```python
from build123d import *

# Parameters (mm, degrees)
F0_W     = 355.6
F0_H     = 355.6
F1_DEPTH = 12.7
F2_W     = 355.6
F2_H     = 12.7
F4_DEPTH = 101.6
F5_W     = 330.2
F5_H     = 12.7
F6_DEPTH = 101.6


with BuildPart() as f1:
    # F0 (on Top) → F1 (new body)
    with BuildSketch(Plane.XY):
        Rectangle(F0_W, F0_H)
    extrude(amount=F1_DEPTH)

    # F2 (on face) + F3 (on face) → F4 (join)
    with BuildSketch(Plane.XY.offset(12.7)):
        with Locations((0, 171.45)):
            Rectangle(F2_W, F2_H)
    with BuildSketch(Plane.XY.offset(12.7)):
        Polygon((-165.1, -177.8), (-165.1, 177.8), (-177.8, 177.8), (-177.8, -165.1), (-177.8, -177.8), align=None)
        Polygon((177.8, -177.8), (177.8, 165.1), (165.1, 165.1), (165.1, -165.1), (165.1, -177.8), align=None)
    extrude(amount=F4_DEPTH)

    # F5 (on face) → F6 (join)
    with BuildSketch(Plane.XY.offset(12.7)):
        with Locations((0, -171.45)):
            Rectangle(F5_W, F5_H)
    extrude(amount=F6_DEPTH)


solid = f1.part
```
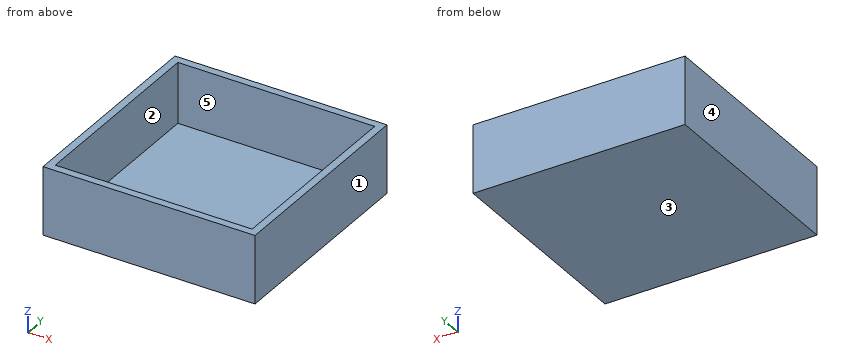
Input: part model. Units: mm. Frame: model coordinates. Face numbers are marked on the shaded views. A direction names the side the tool comes from. Round coordinates to 2 decimals unless told otherwise and drop trailing zeros. Write each loop counter-clockwise with the first axis right and the second up, starting at its lowest first coordinate (ties: lowest second). Pieces come first, ordered by that corner, then holes. Notation, with made-up numbers: (46, 69.5) -> (83, 69.5) arc R17 ccw to (83, 78.5) -> close; hole circle Ø11 at (-1.5, -18). An arc over 180 degrees is marked (long way). Answer as CSV lines item,"result".
1. Ray query, L1, parallel to X at y = -126.5, z = 64; L2, parallel to Z at x = -22.5, y = -44.5. Return the intervals inside material, ascending. Write a range as [from, to].
Geometry says:
L1,"x = [-177.8, -165.1], [165.1, 177.8]"
L2,"z = [0, 12.7]"
2. Reachability of the marked faces 4 and 5 from +Z, -Z, +X, -X, +Y, -Y: full face, straight path, thin tool, end or side. Return the list, or none.
Geometry says:
face 4,"+Z, -Z, -X, +Y, -Y"
face 5,"+Z"
3. Section B-B (y = 84). Return the cut outline in (x, z).
Geometry says:
outline,"(-177.8, 0) -> (177.8, 0) -> (177.8, 114.3) -> (165.1, 114.3) -> (165.1, 12.7) -> (-165.1, 12.7) -> (-165.1, 114.3) -> (-177.8, 114.3) -> close"
4. Section A-A (z = 51.5). Return the cut outline in (x, y).
Geometry says:
outline,"(-177.8, -177.8) -> (177.8, -177.8) -> (177.8, 177.8) -> (-177.8, 177.8) -> close; hole (-165.1, -165.1) -> (165.1, -165.1) -> (165.1, 165.1) -> (-165.1, 165.1) -> close"
5. Mould query, pull axis X, two halves, no side actions, for the marked faces 1, 2 and 3. Classes: +X half, -X half, draft (parallel to the pull), parting line (faces both ways), or undercut.
Geometry says:
face 1,"+X half"
face 2,"undercut"
face 3,"draft"
6. Contact query for a flat-ended pin moving along its axis: P1, Ø4, axis at x = 90, y = 90.5, coming from the +Z side. Output: stop coordinate, or through.
Geometry says:
P1,"stops at z = 12.7"
